Verification items for this drawing (mm, ordinates from the low corner). A direction names the side the tool comes from. Coordinates: 2 decimals unless noted, no trailing zeros. Order: outer loops, then holes, each group sorted by start corner. A loop starts at its lowest first (then second) coordinate and runs counter-clockwise, first axis right, second up.
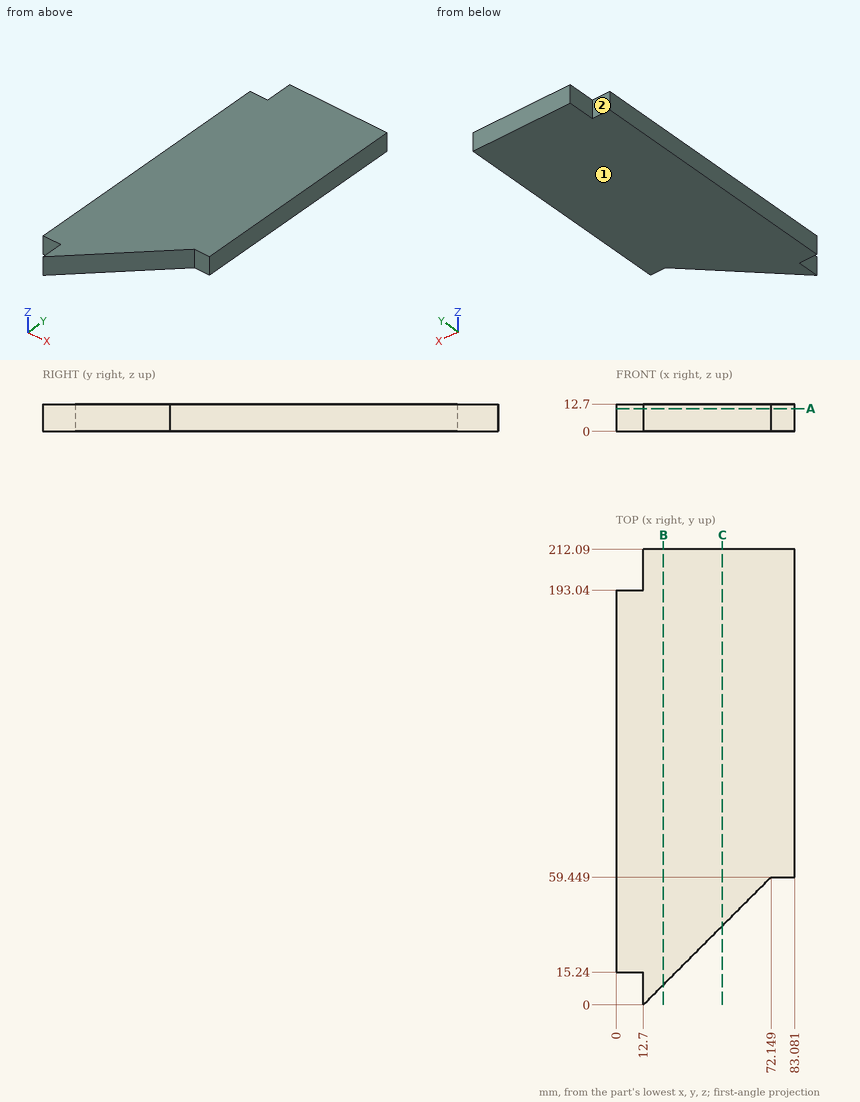
(1) Cross-section at C-C (x = 49.5). Enter the section's corners in (y, z), and give its area (3 significant figures).
Filled in:
outline: (36.8, 0) - (212.09, 0) - (212.09, 12.7) - (36.8, 12.7) - close
area: 2,230 mm2
(2) Cross-section at A-A (z = 10.5). Enter the section's corners in (x, y), and give its area (3 significant figures).
Filled in:
outline: (0, 15.24) - (12.7, 15.24) - (12.7, 0) - (72.15, 59.45) - (83.08, 59.45) - (83.08, 212.09) - (12.7, 212.09) - (12.7, 193.04) - (0, 193.04) - close
area: 14,800 mm2
(3) Cross-section at B-B (x = 22). Enter the section's corners in (y, z).
Filled in:
outline: (9.3, 0) - (212.09, 0) - (212.09, 12.7) - (9.3, 12.7) - close
(4) Thickness scan on probe 1 along Y at (x, z) = (78.5, 11); probe 2 along Y at (x, z) = (12.5, 5); probe 3 along X at (y, z) = (52, 9.5). Record the ranges inside material, lowest first.
Filled in:
probe 1: y = 59.45 to 212.09
probe 2: y = 15.24 to 193.04
probe 3: x = 0 to 64.7
(5) Tool access check on the marked faces 1 and 2. Record the directions out of +Z, -Z, +X, -X, +Y, -Y that give a thin tool (end or side, any length) a straight path to the whole face; none if there is none.
Filled in:
face 1: -Z, +X, -X, +Y, -Y
face 2: +Z, -Z, -X, +Y
(6) Go/stop test with flat-tipped pins: P1, Ø6.5, axis at y = 201, z = 8.5, coming from the -X side; P2, Ø6.5, axis at x = 6.5, z = 6, coming from the -Y side; P3, Ø1.5, axis at x = 26, z = 7.5, coming from the -Y side; P4, Ø12, axis at x = 61, y = 31.5, coming from the +Z side. Record where each tip stops, or that it passes through.
Filled in:
P1: stops at x = 12.7
P2: stops at y = 15.24
P3: stops at y = 12.55
P4: passes through
